from build123d import *

# Parameters (mm, degrees)
F_0105_CYLINDER_SKETCH_R    = 3.25
F_0105_CYLINDER_DEPTH       = 2.5
F_0106_FILLET_R             = 0.625
F_0107_EXTRUDE_DEPTH        = 1.385
F_0107_EXTRUDE_ROTATE_ANGLE = 120
F_0110_CYLINDER_SKETCH_R    = 1.2
F_0110_CYLINDER_DEPTH       = 24.7
F_0111_CONE_ROTATE_ANGLE    = 90


with BuildPart() as part:
    # 0105_cylinder_Sketch → 0105_cylinder (new body)
    with BuildSketch(Plane.XY):
        Circle(F_0105_CYLINDER_SKETCH_R)
    extrude(amount=F_0105_CYLINDER_DEPTH)

    # 0106_fillet
    f_0106_fillet_edges = [part.edges().sort_by_distance(p)[0] for p in [
        (-3.25, 0, 2.5),
    ]]
    fillet(f_0106_fillet_edges, radius=F_0106_FILLET_R)


with BuildPart() as body_2:
    # 0107_extrude_Sketch → 0107_extrude (new body)
    with BuildSketch(Plane.XY):
        Polygon((0, 0), (1.154700538, 0), (1.732050808, 1), (1.154700538, 2), (0, 2), (-0.577350269, 1), align=None)
    extrude(amount=F_0107_EXTRUDE_DEPTH)


with BuildPart() as body_2_1:
    # 0107_extrude_Rotate: read off the stored shape, not the designer's step
    # 0107_extrude_Rotate: moved
    add(body_2.part.rotate(Axis((0, 0, 0), (0, 0, 1)), F_0107_EXTRUDE_ROTATE_ANGLE))


with BuildPart() as body_2_2:
    # 0107_extrude_Translate: moved
    add(body_2_1.part.moved(Location((1.154700538, 0, 1.125))))


with BuildPart() as part_1:
    add(part.part)

    # 0109_sub: cut body 2
    add(body_2_2.part, mode=Mode.SUBTRACT)


with BuildPart() as body_2_2_1:
    # 0110_cylinder_Sketch → 0110_cylinder (new body)
    with BuildSketch(Plane.XY):
        Circle(F_0110_CYLINDER_SKETCH_R)
    extrude(amount=F_0110_CYLINDER_DEPTH)


with BuildPart() as body_2_2_2:
    # 0110_cylinder_Translate: moved
    add(body_2_2_1.part.moved(Location((0, 0, -24.7))))


with BuildPart() as body_3:
    # 0111_cone_Sketch → 0111_cone (revolve)
    with BuildSketch(Plane.XY, mode=Mode.PRIVATE) as f_0111_cone_sk:
        Polygon((0, 0), (1.2, 0), (0.9, 0.3), (0, 0.3), align=None)
    revolve(f_0111_cone_sk.sketch.rotate(Axis((0, -100, 0), (0, 1, 0)), 90), axis=Axis((0, -100, 0), (0, 1, 0)))


with BuildPart() as body_3_1:
    # 0111_cone_Rotate: moved
    add(body_3.part.rotate(Axis((0, 0, 0), (1, 0, 0)), F_0111_CONE_ROTATE_ANGLE))


with BuildPart() as body_3_2:
    # 0111_cone_Translate: moved
    add(body_3_1.part.moved(Location((0, 0, -25))))


with BuildPart() as body_2_2_3:
    add(body_2_2_2.part)

    # 0113_add: union body 3
    add(body_3_2.part)


with BuildPart() as part_2:
    add(part_1.part)

    # 0114_add: union body 2 2
    add(body_2_2_3.part)


solid = part_2.part
Part model, mm, in its own coordinate system. A direction names the side the tool comes from. Give positions to 0.01 mm unless a question says otherwise; leave off trailing zeros. Loops run counter-clockwise (first coordinate to the right, second up) from the corner with the lowest first, then second, coordinate; pieces in that order, holes last. Notation, with made-up numbers: (66.25, 36.25) -> (93.25, 36.25) arc R28 cw to (93.25, 60.25) -> close; hole circle Ø7 at (-34, 42.25). An arc over 180 degrees is marked (long way). Write each question's results on one line, items separated by ' | '. Start each with the question number.
Q1. Which spindle directions (+Z, -Z, +X, -X, +Y, -Y) get a long thin tool onto all of the face, cutting with end or side? Do faces 4 (the face through (-0.87, -0.49, 1.8)), 5 (the face through (-2.579, -1.978, 0.924)), 6 (the face through (1.4, 0, 0)). Say none if no direction does.
Q2. Pull direction Y, two halves, no side cores. Call faces 1 (the face through (-0.86, 0.51, 1.8)), 2 (the face through (0, 0, -25)), 3 (the face through (0.65, 1.01, -12.52)): +Y half, -Y half, draft (parallel to the pull), parting line (faces both ways), or undercut.
Q3. Band-saw the part on B-B on z = -10.25. List the corners of the cut face in (x, y).
Q4. Band-saw the part on A-A on x = 0. List the corners of the cut face in (y, z) (3 decimals), plus the area to 3 significant figures.
Q5. Pin check, flat tips, straight feed: P1, Ø0.6, axis at x = -0.5, y = 0, coming from the +Z side (3 decimals); P2, Ø1, axis at x = 0, z = -7, coming from the +Y side; P3, Ø1.5, axis at x = 2.5, z = -20, coming from the +Y side; P4, Ø2, axis at x = -1, z = -7, coming from the -Y side. Stop position of each tip, or through.
Q6. Wall check: L1, parallel to Z at x = -1, y = 0.75; L2, parallel to Y at x = 0, z = -10; L3, parallel to Z at x = -2.25, y = -2.25. Give the ranges that are in metal, low to high.
Results are:
1) face 4: +Z | face 5: +Z, -Z | face 6: -Z
2) face 1: undercut | face 2: draft | face 3: parting line
3) outline: circle Ø2.4 at (0, 0)
4) outline: (-3.25, 0) -> (-1.2, 0) -> (-1.2, -24.7) -> (-0.9, -24.7) -> (-1.2, -25) -> (1.2, -25) -> (0.9, -24.7) -> (1.2, -24.7) -> (1.2, 0) -> (3.25, 0) -> (3.25, 1.875) arc R0.625 ccw to (2.625, 2.5) -> (1, 2.5) -> (1, 1.125) -> (-1, 1.125) -> (-1, 2.5) -> (-2.625, 2.5) arc R0.625 ccw to (-3.25, 1.875) -> close | area: 73.2 mm²
5) P1: stops at z = 1.125 | P2: stops at y = 1.2 | P3: passes through | P4: stops at y = -1.2
6) L1: z = 0 to 2.5 | L2: y = -1.2 to 1.2 | L3: z = 0 to 2.16
